from build123d import *

# Parameters (mm, degrees)
SKETCH1_R               = 2.1
BOSS_EXTRUDE2_DEPTH     = 3
SKETCH1_14_R            = 5
CUT_EXTRUDE2_DEPTH      = 10
SKETCH2_R               = 2
SKETCH2_W               = 15
SKETCH2_H               = 4
SKETCH2_R_2             = 3.9
BOSS_EXTRUDE3_DEPTH     = 7
SKETCH2_4_R             = 3.25
SKETCH2_4_R_2           = 3.3
CUT_EXTRUDE3_DEPTH      = 7
CUT_EXTRUDE4_DEPTH      = 61.199667773
CUT_EXTRUDE4_DEPTH_BACK = 7
SKETCH3_R               = 1
FILLET1_R               = 12
CUT_EXTRUDE5_START      = -41
SKETCH3_3_R             = 1
CUT_EXTRUDE5_DEPTH      = 9


with BuildPart() as part:
    # Sketch1 → Boss-Extrude2 (new body)
    with BuildSketch(Plane(origin=(0, 0, 0), x_dir=(1, 0, 0), z_dir=(0, 1, 0))):
        with BuildLine():
            Line((32, -25), (32, -14.320549047))
            Line((32, -14.320549047), (28.692414075, -11.736497543))
            ThreePointArc((28.692414075, -11.736497543), (31, 0), (28.692414075, 11.736497543))
            Line((28.692414075, 11.736497543), (32, 14.320549047))
            Line((32, 14.320549047), (32, 25))
            Line((32, 25), (-32, 25))
            Line((-32, 25), (-32, 14.320549047))
            Line((-32, 14.320549047), (-28.692414075, 11.736497543))
            ThreePointArc((-28.692414075, 11.736497543), (-31, 0), (-28.692414075, -11.736497543))
            Line((-28.692414075, -11.736497543), (-32, -14.320549047))
            Line((-32, -14.320549047), (-32, -25))
            Line((-32, -25), (32, -25))
        make_face()
        with Locations(Location((26, 0, 0), (0, 0, 270))):
            Circle(SKETCH1_R, mode=Mode.SUBTRACT)
        with Locations(Location((-26, 0, 0), (0, 0, 270))):
            Circle(SKETCH1_R, mode=Mode.SUBTRACT)
    extrude(amount=BOSS_EXTRUDE2_DEPTH)

    # Sketch1<14> → Cut-Extrude2 (cut)
    with BuildSketch(Plane(origin=(0, 0, 0), x_dir=(1, 0, 0), z_dir=(0, 1, 0))):
        with Locations(Location((0, 0, 0), (0, 0, 270))):
            Circle(SKETCH1_14_R)
    extrude(amount=CUT_EXTRUDE2_DEPTH, mode=Mode.SUBTRACT)

    # Sketch2 → Boss-Extrude3 (add)
    with BuildSketch(Plane(origin=(0, 3, 0), x_dir=(1, 0, 0), z_dir=(0, 1, 0))):
        with Locations(Location((10.75, -10, 0), (0, 0, 269.999999999))):
            Circle(SKETCH2_R)
        Polygon((8.75, -21), (1.25, -21), (1.25, -25), (16.25, -25), (16.25, -21), align=None)
        with Locations((8.75, 23)):
            Rectangle(SKETCH2_W, SKETCH2_H)
        with Locations(Location((19.75, 0, 0), (0, 0, 270))):
            Circle(SKETCH2_R_2)
        with Locations(Location((10.75, 10, 0), (0, 0, 270))):
            Circle(SKETCH2_R)
    extrude(amount=BOSS_EXTRUDE3_DEPTH)

    # Sketch2<4> → Cut-Extrude3 (cut)
    with BuildSketch(Plane(origin=(0, 3, 0), x_dir=(1, 0, 0), z_dir=(0, 1, 0))):
        with Locations(Location((12, 17.5, 0), (0, 0, 270))):
            Circle(SKETCH2_4_R)
        with Locations(Location((4.7, 12, 0), (0, 0, 270))):
            Circle(SKETCH2_4_R_2)
        with Locations(Location((12, -17.5, 0), (0, 0, 270))):
            Circle(SKETCH2_4_R)
        with Locations(Location((4.7, -12, 0), (0, 0, 270))):
            Circle(SKETCH2_4_R_2)
    extrude(amount=-CUT_EXTRUDE3_DEPTH, mode=Mode.SUBTRACT)

    # Sketch3 → Cut-Extrude4 (cut, two sides: drawn at the far end of the back side and taken through both)
    with BuildSketch(Plane.XY.offset(25).offset(-CUT_EXTRUDE4_DEPTH_BACK)):
        with Locations(Location((8.5, 6, 0), (0, 0, 180))):
            Circle(SKETCH3_R)
    extrude(amount=CUT_EXTRUDE4_DEPTH + CUT_EXTRUDE4_DEPTH_BACK, mode=Mode.SUBTRACT)

    # Fillet1
    # the kernel refuses this fillet: 12 mm, written as the material it takes off along each edge
    with BuildSketch(Plane(origin=(1.25, 10, -52.271780287), x_dir=(0, -1, 0), z_dir=(0, 0, 1)), Plane(origin=(16.25, 10, -21), x_dir=(0, -1, 0), z_dir=(0, 0, -1)), Plane(origin=(1.25, 10, 21), x_dir=(0, -1, 0), z_dir=(0, 0, 1)), Plane(origin=(16.25, 10, 52.271780287), x_dir=(0, -1, 0), z_dir=(0, 0, -1))) as fillet1_piece_1:
        with BuildLine():
            CenterArc((12, 10.908712115), FILLET1_R, 180, 65.375681648)
            Line((0, 10.908712115), (0, 0))
            Line((0, 0), (7, 0))
        make_face()
    extrude(amount=31.271780287, mode=Mode.SUBTRACT)

    # Sketch3<3> → Cut-Extrude5 (cut)
    with BuildSketch(Plane.XY.offset(25).offset(CUT_EXTRUDE5_START)):
        with Locations(Location((8.5, 6, 0), (0, 0, 180))):
            Circle(SKETCH3_3_R)
    extrude(amount=-CUT_EXTRUDE5_DEPTH, mode=Mode.SUBTRACT)


solid = part.part
Design review of the part built by this model. Coordinates are the model's own, in mm. A direction names the side the tool comes from. Coordinates: 2 decimals unless noted, no trailing zeros. Loops run counter-clockwise (first coordinate to the right, second up) from the corner with the lowest first, then second, coordinate; pieces in that order, holes last. Notation, with made-up numbers: (7, -14.75) -> (46, -14.75) arc R12 cw to (46, 4.25) -> close; hole circle Ø2 at (19, 61.25). An arc over 180 degrees is marked (long way). Use a Markdown table: item, result. Add a question column.
Item 1: We need section C-C, the plane x = 10.75. Write out the cut boundary in (y, z).
Item 2: Wall thickness on L1, parallel to Z at x = 0, y = 2.25; L2, parallel to Z at x = 4.5, y = 5.5; L3, parallel to X at y = 1.3, z = -17.5: over which ranges is each line inside the solid? List them lowest first. Write a range as from..to.
Item 3: We need section B-B, the plane y = 1.5. Write out the cut boundary in (x, z), and give its area (3 significant figures).
Item 4: Machinability: for faces 4 (the cylindrical face through (12.733, 6.451, -10.26)), 5 (the flat face through (8.6, 4.8, -21)), 6 (the flat face through (11, 10, 10)), 7 (the cylindrical face through (9.237, 5.324, 22.972)), which of the approach directions +Z, -Z, +X, -X, +Y, -Y give a long, thin tool a straight path to every point of the face, cutting with its end or side? Answer none if there is none.
Item 5: Clearance check with flat-ended pins moving along their axes: P1, Ø5, axis at x = 9, z = -15, coming from the -Y side; P2, Ø8, axis at x = 5.5, z = 4, coming from the +Y side; P3, Ø1.6, axis at x = 8.5, y = 6, coming from the -Z side; P4, Ø6, axis at y = 8.5, z = 13, coming from the -X side. State where each tip first meets the part, or that it passes through.
Item 6: We need section A-A, the plane z = 0. Write out the cut boundary in (x, y).
Item 7: The part is to be moulded in two halves that separate along Y. For faces 1 (the cylindrical face through (9.237, 5.324, -22.972)), 2 (the cylindrical face through (13.15, 7.11, -22.97)), 3 (the flat face through (30.369, 1.479, 13.047)), say which applies: +Y half, -Y half, draft (parallel to the pull), parting line (faces both ways), or undercut.
Item 8: We need section D-D, the plane x = 0. Write out the cut boundary in (y, z), and give its area (3 significant figures).
Numbers:
| question | item | result |
|---|---|---|
| 1 | outline | (0, -25) -> (8.71, -25) -> (8.71, -21) -> (3, -21) -> (3, -20.5) -> (0, -20.5) -> close; (0, -14.5) -> (3, -14.5) -> (3, -12) -> (10, -12) -> (10, -8) -> (3, -8) -> (3, 8) -> (10, 8) -> (10, 12) -> (3, 12) -> (3, 14.5) -> (0, 14.5) -> close; (0, 20.5) -> (3, 20.5) -> (3, 21) -> (8.71, 21) -> (8.71, 25) -> (0, 25) -> close |
| 2 | L1 | z = -25..-5, 5..25 |
| 2 | L2 | z = -25..-21, 21..25 |
| 2 | L3 | x = -32..8.75, 15.25..32 |
| 3 | outline | (-32, -25) -> (32, -25) -> (32, -14.32) -> (28.69, -11.74) arc R31 ccw to (28.69, 11.74) -> (32, 14.32) -> (32, 25) -> (-32, 25) -> (-32, 14.32) -> (-28.69, 11.74) arc R31 ccw to (-28.69, -11.74) -> (-32, -14.32) -> close; hole circle Ø4.2 at (-26, 0); hole circle Ø10 at (0, 0); hole circle Ø6.6 at (4.7, -12); hole circle Ø6.6 at (4.7, 12); hole circle Ø6.5 at (12, -17.5); hole circle Ø6.5 at (12, 17.5); hole circle Ø4.2 at (26, 0) |
| 3 | area | 2,860 mm^2 |
| 4 | face 4 | +Y |
| 4 | face 5 | +X, -X, +Y |
| 4 | face 6 | +Z, -Z, +X, -X, +Y |
| 4 | face 7 | +Z |
| 5 | P1 | stops at y = 0 |
| 5 | P2 | stops at y = 3 |
| 5 | P3 | stops at z = -11.38 |
| 5 | P4 | stops at x = 8.75 |
| 6 | outline | (-31, 0) -> (-28.1, 0) -> (-28.1, 3) -> (-31, 3) -> close; (-23.9, 0) -> (-5, 0) -> (-5, 3) -> (-23.9, 3) -> close; (5, 0) -> (23.9, 0) -> (23.9, 3) -> (23.65, 3) -> (23.65, 10) -> (15.85, 10) -> (15.85, 3) -> (5, 3) -> close; (28.1, 0) -> (31, 0) -> (31, 3) -> (28.1, 3) -> close |
| 7 | face 1 | undercut |
| 7 | face 2 | +Y half |
| 7 | face 3 | draft |
| 8 | outline | (0, -25) -> (3, -25) -> (3, -5) -> (0, -5) -> close; (0, 5) -> (3, 5) -> (3, 25) -> (0, 25) -> close |
| 8 | area | 120 mm^2 |
